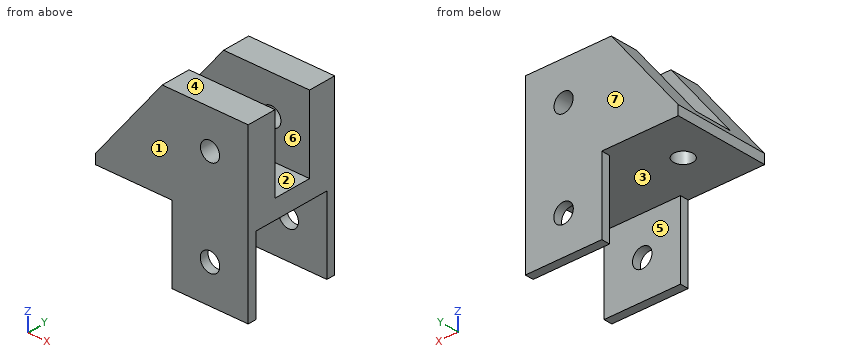
```python
from build123d import *

# Parameters (mm, degrees)
SKETCH2_W           = 20
SKETCH2_H           = 5
SKETCH2_H_2         = 5.5
BOSS_EXTRUDE1_DEPTH = 20
SKETCH3_R           = 2.5
SKETCH3_R_2         = 2.55
CUT_EXTRUDE1_DEPTH  = 56.226805086
BOSS_EXTRUDE2_DEPTH = 20
CUT_EXTRUDE2_DEPTH  = 56.226805086
SKETCH7_R           = 2.55
CUT_EXTRUDE3_DEPTH  = 20


with BuildPart() as part:
    # Sketch2 → Boss-Extrude1 (new body)
    with BuildSketch(Plane(origin=(0, 0, 0), x_dir=(0, 0, -1), z_dir=(1, 0, 0))):
        Polygon((20, 7.75), (20, 2.25), (25, 2.25), (25, 22.75), (20, 22.75), (20, 17.75), align=None)
        Polygon((25, 22.75), (45, 22.75), (45, 25), (0, 25), (0, 22.75), (20, 22.75), align=None)
        Polygon((0, 2.25), (0, 0), (45, 0), (45, 2.25), (25, 2.25), (20, 2.25), align=None)
        with Locations((10, 20.25)):
            Rectangle(SKETCH2_W, SKETCH2_H)
        with Locations((10, 5)):
            Rectangle(SKETCH2_W, SKETCH2_H_2)
    extrude(amount=BOSS_EXTRUDE1_DEPTH)

    # Sketch3 → Cut-Extrude1 (cut, through all)
    with BuildSketch(Plane(origin=(0, 25, 0), x_dir=(1, 0, 0), z_dir=(0, 1, 0))):
        with Locations(Location((10, 10, 0), (0, 0, 270))):
            Circle(SKETCH3_R)
        with Locations(Location((10, 35, 0), (0, 0, 270))):
            Circle(SKETCH3_R_2)
    extrude(amount=-CUT_EXTRUDE1_DEPTH, mode=Mode.SUBTRACT)

    # Sketch5 → Boss-Extrude2 (add)
    with BuildSketch(Plane.ZY):
        Polygon((-25, 25), (-25, 22.75), (-25, 2.25), (-25, 0), (0, 0), (0, 7.75), (-20, 7.75), (-20, 17.75), (0, 17.75), (0, 25), align=None)
    extrude(amount=BOSS_EXTRUDE2_DEPTH)

    # Sketch6 → Cut-Extrude2 (cut, through all)
    with BuildSketch(Plane.XZ):
        Polygon((-20, -22.5), (-2.5, 0), (-20, 0), align=None)
    extrude(amount=-CUT_EXTRUDE2_DEPTH, mode=Mode.SUBTRACT)

    # Sketch7 → Cut-Extrude3 (cut)
    with BuildSketch(Plane.XY.offset(-20)):
        with Locations((-10, 12.5)):
            Circle(SKETCH7_R)
    extrude(amount=-CUT_EXTRUDE3_DEPTH, mode=Mode.SUBTRACT)


solid = part.part
```
Design review of the part built by this model. Coordinates are the model's own, in mm. Face numbers are marked on the shaded views. A direction names the side the tool comes from. Coordinates: 2 decimals unless noted, no trailing zeros. Write each loop counter-clockwise with the first axis right and the second up, starting at its lowest first coordinate (ties: lowest second). Pieces come first, ordered by that corner, then holes.
1) Add section C-C (y = 11.25). Write out the cut boundary in (x, z), plus the area to 3 significant figures.
2) To check wall thickness, follow L1, parallel to X at y = 0.95, z = -35; L2, parallel to Y at x = 7.5, z = -40; L3, parallel to Y at x = -10, z = -17.5. State the ranges of each line that lie inside material, in increasing order.
3) Insertion check: pin 1 (5 mm diameter, centred on x = 8, y = 10.5, fed in from +Z); pin 2 (2 mm diameter, centred on x = -12.5, y = 16, fed in from -Z); pin 3 (5 mm diameter, centred on x = 5, z = -23.5, fed in from -Y); pin 4 (1.1 mm diameter, centred on y = 0.5, z = -35.5, fed in from -X). Each pin has a flat end and moves straight along its axis. Give the tip position at first contact, or say it passes through.
4) Add section A-A (z = -39). Write out the cut boundary in (x, y), plus the area to 3 significant figures.
5) Add section D-D (x = -11). Write out the cut boundary in (y, z).
6) Machinability: for the marked faces 5, 6 and 7, which of the approach directions +Z, -Z, +X, -X, +Y, -Y give a long, thin tool a straight path to every point of the face, cutting with its end or side? Answer none if there is none.
7) Add section B-B (x = 10). Write out the cut boundary in (y, z).
8) Mouldability with a two-part tool opening along Y and no side actions: class the marked faces 1, 2, 3 and 4 as +Y half, -Y half, draft (parallel to the pull), parting line (faces both ways), or undercut.
Check result:
1. outline: (-20, -25) - (-12.22, -25) - (-12.22, -20) - (-18.06, -20) - (-20, -22.5) - close; (-7.78, -25) - (20, -25) - (20, -20) - (-7.78, -20) - close
1. area: 175 mm2
2. L1: x = 0 to 7.45, 12.55 to 20
2. L2: y = 0 to 2.25, 22.75 to 25
2. L3: y = 0 to 7.75, 17.75 to 25
3. pin 1: stops at z = -20
3. pin 2: stops at z = -25
3. pin 3: stops at y = 0
3. pin 4: stops at x = 0
4. outline: (0, 0) - (20, 0) - (20, 2.25) - (0, 2.25) - close; (0, 22.75) - (20, 22.75) - (20, 25) - (0, 25) - close
4. area: 90.0 mm2
5. outline: (0, -25) - (10.15, -25) - (10.15, -20) - (7.75, -20) - (7.75, -10.93) - (0, -10.93) - close; (14.85, -25) - (25, -25) - (25, -10.93) - (17.75, -10.93) - (17.75, -20) - (14.85, -20) - close
6. face 5: -Z, +X, -X
6. face 6: +Z, +X, -X
6. face 7: +Z, -Z, +X, -X, +Y
7. outline: (0, -45) - (2.25, -45) - (2.25, -37.55) - (0, -37.55) - close; (0, -32.45) - (2.25, -32.45) - (2.25, -25) - (22.75, -25) - (22.75, -32.45) - (25, -32.45) - (25, -12.5) - (17.75, -12.5) - (17.75, -20) - (7.75, -20) - (7.75, -12.5) - (0, -12.5) - close; (0, -7.5) - (7.75, -7.5) - (7.75, 0) - (0, 0) - close; (17.75, -7.5) - (25, -7.5) - (25, 0) - (17.75, 0) - close; (22.75, -45) - (25, -45) - (25, -37.55) - (22.75, -37.55) - close
8. face 1: -Y half
8. face 2: undercut
8. face 3: undercut
8. face 4: draft
